Geometry check sheet. Reference: the model listing, model coordinates, mm. A direction names the side the tool comes from. Round coordinates to 2 decimals unless told otherwise and drop trailing zeros. Loops run counter-clockwise (first coordinate to the right, second up) from the corner with the lowest first, then second, coordinate; pieces in that order, holes last. Notation, with made-up numbers: (5, -17.5) -> (52, -17.5) arc R24 cw to (52, -7.5) -> close; hole circle Ø5 at (74, 2.25). An arc over 180 degrees is marked (long way). Use a Markdown table: item, result. Add a question column.
Q1. Material ranges on L1, parallel to Z at x = -36, y = -1.5; L2, parallel to Y at x = 0, z = 13; L3, parallel to Y at x = 2.5, z = 25.5, recorded low to high.
Q2. Sectioned sample at D-D, the plane y = 63. Enter the section's corners in (x, z), then the cut area to 3 significant figures.
Q3. Sectioned sample at C-C, the plane z = 17. Enter the section's corners in (x, y).
Q4. Gauge pin test, flat ends, axial feed: P1, Ø5, axis at y = 30.5, z = 26.5, coming from the +X side; P2, Ø4, axis at x = -55.5, y = 37.5, coming from the +Z side; P3, Ø8, axis at y = 10.5, z = 15.5, coming from the +X side; P4, Ø6, axis at y = 2.5, z = 32, coming from the -X side. Record the tip position at first contact, or that the pin passes through.
Q5. Set-up check for faces 1 (the face through (-1.172, 8.923, 22.255)), 2 (the face through (-9.764, 74.362, 2.465)): record each of +Z, -Z, +X, -X, +Y, -Y from which the full face is reachable in a straight line by a thin tool's end or side.
Q6. Sectioned sample at A-A, the plane x = 0. Enter the section's corners in (y, z).
```python
from build123d import *

# Parameters (mm, degrees)
F0_R     = 9
F1_DEPTH = 40
F2_R     = 75
F3_DEPTH = 5
F4_R     = 2.5
F5_DEPTH = 25


with BuildPart() as f1:
    # F0 (on Top) → F1 (new body)
    with BuildSketch(Plane.XY):
        Circle(F0_R)
    extrude(amount=F1_DEPTH)

    # F2 (on Top) → F3 (join)
    with BuildSketch(Plane.XY):
        Circle(F2_R)
    extrude(amount=F3_DEPTH)

    # F4 (on face) → F5 (join)
    with BuildSketch(Plane.XY.offset(5)):
        with Locations((-56.467045, 36.209807)):
            Circle(F4_R)
    extrude(amount=F5_DEPTH)


solid = f1.part
```
Values:
| question | item | result |
|---|---|---|
| 1 | L1 | 0 to 5 |
| 1 | L2 | -9 to 9 |
| 1 | L3 | -8.65 to 8.65 |
| 2 | outline | (-40.69, 0) -> (40.69, 0) -> (40.69, 5) -> (-40.69, 5) -> close |
| 2 | area | 407 mm^2 |
| 3 | outline | circle Ø5 at (-56.47, 36.21); circle Ø18 at (0, 0) |
| 4 | P1 | through |
| 4 | P2 | z = 30 |
| 4 | P3 | x = 6.22 |
| 4 | P4 | x = -9 |
| 5 | face 1 | +Z |
| 5 | face 2 | +Z, -Z |
| 6 | outline | (-75, 0) -> (75, 0) -> (75, 5) -> (9, 5) -> (9, 40) -> (-9, 40) -> (-9, 5) -> (-75, 5) -> close |
